Source: CAD feature listing. Evaluate the final solid. Frame: model axes, mm. Round coordinates to 2 decimals unless told otherwise and drop trailing zeros. Loops run counter-clockwise (first coordinate to the right, second up) from the corner with the lowest first, then second, coordinate; pieces in that order, holes last. Notation, with made-up numbers: M -33.75,-22 L -20.75,-22 A21 ccw -20.75,1 Z; hole C 63.5,-1.5 d4. An arc over 180 degrees is marked long. One line per item, written item: value.
from build123d import *

# Parameters (mm, degrees)
SKETCH1_R               = 29.86111111
BOSS_EXTRUDE1_DEPTH     = 1
CUT_EXTRUDE1_DEPTH      = 43.277321503
CUT_EXTRUDE1_DEPTH_BACK = 43.277321503
SKETCH2_R               = 1.25


with BuildPart() as part:
    # Sketch1 → Boss-Extrude1 (new, symmetric)
    with BuildSketch(Plane(origin=(0, 0, 0), x_dir=(1, 0, 0), z_dir=(0, 1, 0))):
        with Locations(Location((0, 0, 0), (0, 0, 270))):
            Circle(SKETCH1_R)
    extrude(amount=BOSS_EXTRUDE1_DEPTH, both=True)

    # Sketch2 → Cut-Extrude1 (cut, two sides: drawn at the far end of the back side and taken through both)
    with BuildSketch(Plane(origin=(0, 1, 0), x_dir=(1, 0, 0), z_dir=(0, 1, 0)).offset(-CUT_EXTRUDE1_DEPTH_BACK)):
        with Locations(Location((1.733610724, -23.686643786, 0), (0, 0, 270))):
            Circle(SKETCH2_R)
        with Locations(Location((-7.46283868, -22.54702949, 0), (0, 0, 270))):
            Circle(SKETCH2_R)
        with Locations(Location((-15.523138546, -17.974834344, 0), (0, 0, 270))):
            Circle(SKETCH2_R)
        with Locations(Location((-21.220181286, -10.66613361, 0), (0, 0, 270))):
            Circle(SKETCH2_R)
        with Locations(Location((-23.686643786, -1.733610724, 0), (0, 0, 270))):
            Circle(SKETCH2_R)
        with Locations(Location((-22.54702949, 7.46283868, 0), (0, 0, 270))):
            Circle(SKETCH2_R)
        with Locations(Location((-17.974834344, 15.523138546, 0), (0, 0, 270))):
            Circle(SKETCH2_R)
        with Locations(Location((-10.66613361, 21.220181286, 0), (0, 0, 270))):
            Circle(SKETCH2_R)
        with Locations(Location((-1.733610724, 23.686643786, 0), (0, 0, 270))):
            Circle(SKETCH2_R)
        with Locations(Location((10.66613361, -21.220181286, 0), (0, 0, 270))):
            Circle(SKETCH2_R)
        with Locations(Location((17.974834344, -15.523138546, 0), (0, 0, 270))):
            Circle(SKETCH2_R)
        with Locations(Location((22.54702949, -7.46283868, 0), (0, 0, 270))):
            Circle(SKETCH2_R)
        with Locations(Location((23.686643786, 1.733610724, 0), (0, 0, 270))):
            Circle(SKETCH2_R)
        with Locations(Location((21.220181286, 10.66613361, 0), (0, 0, 270))):
            Circle(SKETCH2_R)
        with Locations(Location((15.523138546, 17.974834344, 0), (0, 0, 270))):
            Circle(SKETCH2_R)
        with Locations(Location((7.46283868, 22.54702949, 0), (0, 0, 270))):
            Circle(SKETCH2_R)
    extrude(amount=CUT_EXTRUDE1_DEPTH + CUT_EXTRUDE1_DEPTH_BACK, mode=Mode.SUBTRACT)


solid = part.part
1. Section query C-C (z = 16). Return the cut outline in (x, y), and give its area (3 significant figures).
Report:
outline: M -25.21,-1 L 16.82,-1 L 16.82,1 L -25.21,1 Z; M 19.13,-1 L 25.21,-1 L 25.21,1 L 19.13,1 Z
area: 96.2 mm2
2. Ray query, line 1 (X direction, y = -0.85, z = 24.5); line 2 (Z direction, x = 21, y = -0.05); line 3 (X direction, y = 0.6, z = 18). Return the intervals inside material, ascending. Write a range as [from, to].
Report:
line 1: x = [-17.07, 0.78], [2.68, 17.07]
line 2: z = [-21.23, -11.9], [-9.44, 21.23]
line 3: x = [-23.83, -16.77], [-14.27, 23.83]
3. Section query A-A (z = -10.5). Return the cut outline in (x, y), and give its area (3 significant figures).
Report:
outline: M -27.95,-1 L 19.98,-1 L 19.98,1 L -27.95,1 Z; M 22.46,-1 L 27.95,-1 L 27.95,1 L 22.46,1 Z
area: 107 mm2
4. Pull-direction query (X, two-part tool) for faces 1 (the face through (29.607, 0.014, -3.887)), 2 (the face through (0, -1, 0)), 3 (the face through (18.03, -0.014, 14.274)); classes: released by +X, released by -X, zero draft, split by the parting line, or undercut.
Report:
face 1: split by the parting line
face 2: zero draft
face 3: undercut
5. Section query B-B (y = -0.35). Count the separate pieces of the cut face and the enclosed holes in it, and give its area (3 significant figures).
Report:
separate pieces: 1
enclosed holes: 16
area: 2,720 mm2
